from build123d import *

# Parameters (mm, degrees)
F1_DEPTH = 5
F2_R     = 0.9
F3_DEPTH = 50.492125497
F4_DEPTH = 13
F6_DEPTH = 3.3
F8_DEPTH = 1.65
F9_R     = 0.5
F10_R    = 3
F11_R    = 20


with BuildPart() as f1:
    # F0 (on Front) → F1 (new body, symmetric)
    with BuildSketch(Plane.XZ):
        Polygon((15, 30.9), (0, 30.9), (0, 0), (11.6, 0), (11.6, -1.65), (15.76, -1.65), (41.291125497, -19.591125497), (56.541125497, -19.591125497), (56.541125497, -15.441125497), (48.941125497, -15.441125497), (15, 18.5), align=None)
        Polygon((31.8771428741, -10.5313410853), (18.6061007646, -1.2055699989), (31.8771428741, -1.2055699989), align=None, mode=Mode.SUBTRACT)
        with BuildLine():
            Line((33.8771428741, -11.9367727024), (33.8771428741, -3.2055699989))
            Line((33.8771428741, -3.2055699989), (44.405591591, -13.7340187158))
            ThreePointArc((44.405591591, -13.7340187158), (44.6223643423, -14.8238089293), (43.6984848098, -15.441125497))
            Line((43.6984848098, -15.441125497), (39.1802365995, -15.441125497))
            ThreePointArc((39.1802365995, -15.441125497), (38.8787292634, -15.3945893538), (38.6052839044, -15.2593121495))
            Line((38.6052839044, -15.2593121495), (33.8771428741, -11.9367727024))
        make_face(mode=Mode.SUBTRACT)
        with BuildLine():
            Line((29.8771428741, 0.7944300011), (15.76, 0.7944300011))
            Line((15.76, 0.7944300011), (18.2950155817, 10.25523695))
            ThreePointArc((18.2950155817, 10.25523695), (19.0021223629, 10.9623437312), (19.9680481892, 10.7035246861))
            Line((19.9680481892, 10.7035246861), (29.8771428741, 0.7944300011))
        make_face(mode=Mode.SUBTRACT)
    extrude(amount=F1_DEPTH, both=True)

    # F2 (on face) → F3 (cut, through all)
    with BuildSketch(Plane.XY.offset(30.9)):
        with Locations((3, 0)):
            Circle(F2_R)
    extrude(amount=-F3_DEPTH, mode=Mode.SUBTRACT)

    # F2 (on face) → F4 (cut)
    with BuildSketch(Plane.XY.offset(30.9)):
        with Locations((12, 0)):
            Circle(F2_R)
    extrude(amount=-F4_DEPTH, mode=Mode.SUBTRACT)

    # F5 (on face) → F6 (join)
    with BuildSketch(Plane.XY.offset(30.9)):
        with BuildLine():
            Line((7.89, 0.86), (7.11, 0.86))
            ThreePointArc((7.11, 0.86), (6.25, 0), (7.11, -0.86))
            Line((7.11, -0.86), (7.89, -0.86))
            ThreePointArc((7.89, -0.86), (8.75, 0), (7.89, 0.86))
        make_face()
    extrude(amount=F6_DEPTH)

    # F7 (on face) → F8 (join, through all)
    with BuildSketch(Plane(origin=(0, 0, 0), x_dir=(1, 0, 0), z_dir=(0, 0, -1))):
        with BuildLine():
            Line((8.93, -1.035), (8.93, 1.035))
            ThreePointArc((8.93, 1.035), (7.965, 2), (7, 1.035))
            Line((7, 1.035), (7, -1.035))
            ThreePointArc((7, -1.035), (7.965, -2), (8.93, -1.035))
        make_face()
    extrude(amount=F8_DEPTH)

    # F9
    f9_edges = [f1.edges().sort_by_distance(p)[0] for p in [
        (8.75, 0, 34.2),
        (7.5, 0.86, 34.2),
        (6.25, 0, 34.2),
        (7.5, -0.86, 34.2),
        (8.93, 0, -1.65),
        (7.965, -2, -1.65),
        (7, 0, -1.65),
        (7.965, 2, -1.65),
    ]]
    fillet(f9_edges, radius=F9_R)

    # F10
    f10_edges = [f1.edges().sort_by_distance(p)[0] for p in [
        (0, -5, 15.45),
        (0, 5, 15.45),
        (56.541125, -5, -17.516125),
        (56.541125, 5, -17.516125),
    ]]
    fillet(f10_edges, radius=F10_R)

    # F11
    f11_edges = [f1.edges().sort_by_distance(p)[0] for p in [
        (15, 0, 18.5),
    ]]
    fillet(f11_edges, radius=F11_R)


solid = f1.part
Input: part model. Units: mm. Frame: model coordinates. A direction names the side the tool comes from. Round coordinates to 2 decimals unless told otherwise and drop trailing zeros. Order: outer loops, then holes, each group sorted by start corner. A loop starts at its lowest first (then second) coordinate and runs counter-clockwise, first axis right, second up. Notation, with made-up numbers: (-20.75, -10.75) - (28.25, -10.75) arc R16 cw to (28.25, 2.25) - close; hole circle Ø4 at (-35.5, -3.75). An arc over 180 degrees is marked (long way). Answer as a JSON object with one key per item and string values. Group by question number.
(1) Cut plane C-C (y = 3.75). Return loops of the section in (x, z).
(2) Material intervals for probe 1 along Y at (x, z) = (12, 21); probe 2 along X at (y, z) = (4.5, -8.5); probe 3 along X at (y, z) = (1, -8), sorted ascending. Write a range as from..to.
(3) Cut plane B-B (x = 23.5). Return loops of the section in (y, z), then the cut area to 3 significant figures.
(4) Cut plane A-A (z = 26). Return loops of the section in (x, y).
(5) Cut plane D-D (y = -3.25). Return loops of the section in (x, z).
(6) Pin query (flat end, axial travel): P1, Ø3.5, axis at x = 41, y = -2, coming from the +Z side; P2, Ø3, axis at x = 33.5, y = 1.5, coming from the -Z side; P3, Ø4.5, axis at y = 0.5, z = -9, coming from the +X side; P4, Ø1.6, axis at x = 3, y = 0, coming from the -Z side. Return the tip coordinate at first contact, or that it passes through.
(7) Reachability of faces 1 (the face through (41, 0, -15.441)), 2 (the face through (6.25, 0.02, 32.28)), 3 (the face through (11.6, 0, -1)) from +Z, -Z, +X, -X, +Y, -Y: full face, straight path, thin tool, end or side. Return the list, or none.
(8) Draft query along Y for faces 4 (the face through (14, 0, -1.65)), 5 (the face through (0.86, -4.1, 15.23)), 6 (the face through (12, 0, 17.9)). Return one class per face: released by +Y, released by -Y, zero draft, split by the parting line, or undercut.
Here are the results:
{
 "1": {"outline": "(0.56, 0) - (11.6, 0) - (11.6, -1.65) - (15.76, -1.65) - (41.29, -19.59) - (55.98, -19.59) - (55.98, -15.44) - (48.94, -15.44) - (20.86, 12.64) arc R20 cw to (15, 26.78) - (15, 30.9) - (0.56, 30.9) - close; hole (15.76, 0.79) - (29.88, 0.79) - (19.97, 10.7) arc R1 ccw to (18.3, 10.26) - close; hole (18.61, -1.21) - (31.88, -10.53) - (31.88, -1.21) - close; hole (33.88, -11.94) - (38.61, -15.26) arc R1 ccw to (39.18, -15.44) - (43.7, -15.44) arc R1 ccw to (44.41, -13.73) - (33.88, -3.21) - close"},
 "2": {"probe 1": "y = -5..-0.9, 0.9..5", "probe 2": "x = 25.51..28.99, 31.88..33.88, 39.17..42", "probe 3": "x = 24.8..28.27, 31.88..33.88, 38.67..41.5"},
 "3": {"outline": "(-5, -7.09) - (5, -7.09) - (5, -4.64) - (-5, -4.64) - close; (-5, -1.21) - (5, -1.21) - (5, 0.79) - (-5, 0.79) - close; (-5, 7.17) - (5, 7.17) - (5, 10) - (-5, 10) - close", "area": "72.7 mm^2"},
 "4": {"outline": "(0, -2) arc R3 ccw to (3, -5) - (15.02, -5) - (15.02, 5) - (3, 5) arc R3 ccw to (0, 2) - close; hole circle Ø1.8 at (3, 0); hole circle Ø1.8 at (12, 0)"},
 "5": {"outline": "(0.27, 0) - (11.6, 0) - (11.6, -1.65) - (15.76, -1.65) - (41.29, -19.59) - (56.27, -19.59) - (56.27, -15.44) - (48.94, -15.44) - (20.86, 12.64) arc R20 cw to (15, 26.78) - (15, 30.9) - (0.27, 30.9) - close; hole (15.76, 0.79) - (29.88, 0.79) - (19.97, 10.7) arc R1 ccw to (18.3, 10.26) - close; hole (18.61, -1.21) - (31.88, -10.53) - (31.88, -1.21) - close; hole (33.88, -11.94) - (38.61, -15.26) arc R1 ccw to (39.18, -15.44) - (43.7, -15.44) arc R1 ccw to (44.41, -13.73) - (33.88, -3.21) - close"},
 "6": {"P1": "stops at z = -5.75", "P2": "stops at z = -15.17", "P3": "stops at x = 44.75", "P4": "passes through"},
 "7": {"face 1": "+Y, -Y", "face 2": "+Z, -X", "face 3": "-Z, +Y, -Y"},
 "8": {"face 4": "zero draft", "face 5": "released by -Y", "face 6": "undercut"}
}
